Could you check a few things on this model? Use its own coordinates, in mm. Face numbers are marked on the shaded views. A direction names the side the tool comes from. Coordinates: 2 decimals unless noted, no trailing zeros. Loops run counter-clockwise (first coordinate to the right, second up) from the corner with the lowest first, then second, coordinate; pieces in that order, holes last.
1) Imagine slicing it at B-B on y = 5.5. Please give me the cut outline in (x, z), plus the area to 3 significant figures.
2) If I drill on line 1 along Z through (x, y) = (134.75, 45); line 2 along Z through (x, y) = (6.5, 2.5); line 3 along Y through (x, z) = (17, -90.7), over which ranges is the centre line in solid material (lowest first)?
3) Imagine slicing it at D-D on x = 123.5. Please give me the cut outline in (y, z).
4) Thinking about a two-plate mould opening in X: for the marked faces 6, 7 and 8, which applies, released by +X, released by -X, zero draft, split by the parting line, or undercut?
5) For the marked faces 1, 2, 3, 4 and 5, which set-ups out of +Z, -Z, +X, -X, +Y, -Y let a thin tool reach every point of the face, with its end or its side?
6) Will these pins go through, and if not, where does the flat tip stop? P1, Ø5, axis at y = 0.5, z = -75, coming from the -X side; P2, Ø4, axis at x = 12, y = 33.5, coming from the -Z side; P3, Ø13.5, axis at y = 16.5, z = -38.5, coming from the +X side; P4, Ø3, axis at x = -8.75, z = -96.14, coming from the +Y side.
7) Imagine slicing it at C-C on z = -84. Please give me the cut outline in (x, y).
8) Imagine slicing it at A-A on x = 17. Please give me the cut outline in (y, z), plus the area to 4 significant figures.
```python
from build123d import *

# Parameters (mm, degrees)
SKETCH1_W                = 136
SKETCH1_H                = 106
SKETCH1_W_2              = 126
SKETCH1_H_2              = 96
BOSS_EXTRUDE1_DEPTH      = 45
SKETCH2_W                = 136
SKETCH2_H                = 106
BOSS_EXTRUDE3_DEPTH      = 5
SKETCH3_R                = 10.5
CUT_EXTRUDE1_DEPTH       = 5
BOSS_EXTRUDE4_DEPTH      = 5
BOSS_EXTRUDE4_DEPTH_BACK = 5
SKETCH4_W                = 156
SKETCH4_H                = 126
SKETCH4_W_2              = 136
SKETCH4_H_2              = 106
SKETCH5_W                = 136
SKETCH5_H                = 106
SKETCH5_W_2              = 126
SKETCH5_H_2              = 96
BOSS_EXTRUDE6_DEPTH      = 5
CHAMFER1_SIZE            = 5
SKETCH6_R                = 1.75
CUT_EXTRUDE2_DEPTH       = 180.97284412


with BuildPart() as part:
    # Sketch1 → Boss-Extrude1 (new body)
    with BuildSketch(Plane(origin=(0, 0, 0), x_dir=(1, 0, 0), z_dir=(0, 1, 0))):
        with Locations((63, 39.392502756)):
            Rectangle(SKETCH1_W, SKETCH1_H)
        with Locations((63, 39.392502756)):
            Rectangle(SKETCH1_W_2, SKETCH1_H_2, mode=Mode.SUBTRACT)
    extrude(amount=BOSS_EXTRUDE1_DEPTH)

    # Sketch2 → Boss-Extrude3 (add)
    with BuildSketch(Plane.XZ):
        with Locations((63, -39.392502756)):
            Rectangle(SKETCH2_W, SKETCH2_H)
    extrude(amount=BOSS_EXTRUDE3_DEPTH)

    # Sketch3 → Cut-Extrude1 (cut)
    with BuildSketch(Plane.XY.offset(-87.392502756)):
        with Locations((17, 20)):
            Circle(SKETCH3_R)
    extrude(amount=-CUT_EXTRUDE1_DEPTH, mode=Mode.SUBTRACT)

    # Sketch4 → Boss-Extrude4 (add, two sides: drawn at the far end of the back side and taken through both)
    with BuildSketch(Plane(origin=(0, 45, 0), x_dir=(1, 0, 0), z_dir=(0, 1, 0)).offset(-BOSS_EXTRUDE4_DEPTH_BACK)):
        with Locations((63, 39.392502756)):
            Rectangle(SKETCH4_W, SKETCH4_H)
        with Locations((63, 39.392502756)):
            Rectangle(SKETCH4_W_2, SKETCH4_H_2, mode=Mode.SUBTRACT)
    extrude(amount=BOSS_EXTRUDE4_DEPTH + BOSS_EXTRUDE4_DEPTH_BACK)

    # Sketch5 → Boss-Extrude6 (add)
    with BuildSketch(Plane(origin=(0, 45, 0), x_dir=(1, 0, 0), z_dir=(0, 1, 0))):
        with Locations((63, 39.392502756)):
            Rectangle(SKETCH5_W, SKETCH5_H)
        with Locations((63, 39.392502756)):
            Rectangle(SKETCH5_W_2, SKETCH5_H_2, mode=Mode.SUBTRACT)
    extrude(amount=BOSS_EXTRUDE6_DEPTH)

    # Chamfer1
    chamfer1_edges = [part.edges().sort_by_distance(p)[0] for p in [
        (-15, 45, 23.607497244),
        (-15, 45, -102.392502756),
        (141, 45, -102.392502756),
        (141, 45, 23.607497244),
    ]]
    chamfer(chamfer1_edges, length=CHAMFER1_SIZE)

    # Sketch6 → Cut-Extrude2 (cut, through all)
    with BuildSketch(Plane.XZ.offset(-40)):
        with Locations(Location((-8.75, 17.357497244, 0), (0, 0, 270))):
            Circle(SKETCH6_R)
        with Locations(Location((-8.75, -96.142502756, 0), (0, 0, 90))):
            Circle(SKETCH6_R)
        with Locations(Location((134.75, -96.142502756, 0), (0, 0, 270))):
            Circle(SKETCH6_R)
        with Locations(Location((134.75, 17.357497244, 0), (0, 0, 90))):
            Circle(SKETCH6_R)
    extrude(amount=-CUT_EXTRUDE2_DEPTH, mode=Mode.SUBTRACT)


solid = part.part
```
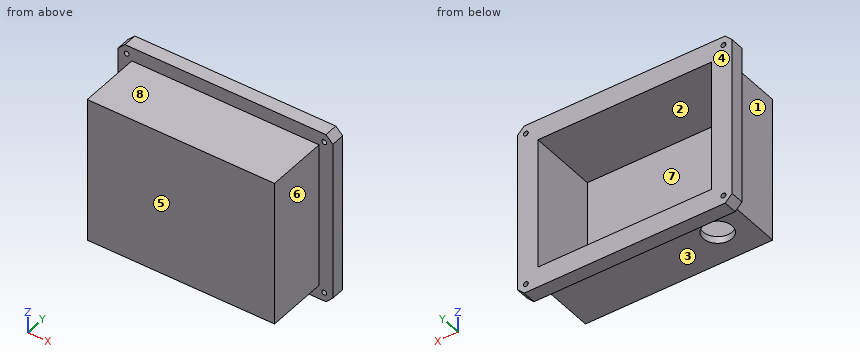
Filled in:
1. outline: (-5, -92.39) - (131, -92.39) - (131, 13.61) - (-5, 13.61) - close; hole (0, -87.39) - (126, -87.39) - (126, 8.61) - (0, 8.61) - close
1. area: 2,320 mm2
2. line 1: z = -102.39 to -97.89, -94.39 to 15.61, 19.11 to 23.61
2. line 2: z = -92.39 to -87.39, 8.61 to 13.61
2. line 3: y = -5 to 9.5, 30.5 to 50
3. outline: (-5, -92.39) - (40, -92.39) - (40, -102.39) - (50, -102.39) - (50, -87.39) - (0, -87.39) - (0, 8.61) - (50, 8.61) - (50, 23.61) - (40, 23.61) - (40, 13.61) - (-5, 13.61) - close
4. face 6: released by +X
4. face 7: undercut
4. face 8: zero draft
5. face 1: +Z, -Z, -X, -Y
5. face 2: +Y
5. face 3: -Z, +X, -X, -Y
5. face 4: +Z, -Z, +X, -X, +Y
5. face 5: +Z, -Z, +X, -X, -Y
6. P1: stops at x = -5
6. P2: stops at z = -92.39
6. P3: stops at x = 131
6. P4: passes through
7. outline: (-15, 40) - (-5, 40) - (-5, -5) - (131, -5) - (131, 40) - (141, 40) - (141, 50) - (126, 50) - (126, 0) - (0, 0) - (0, 50) - (-15, 50) - close
8. outline: (-5, -92.39) - (9.5, -92.39) - (9.5, -87.39) - (0, -87.39) - (0, 8.61) - (50, 8.61) - (50, 23.61) - (40, 23.61) - (40, 13.61) - (-5, 13.61) - close; (30.5, -92.39) - (40, -92.39) - (40, -102.39) - (50, -102.39) - (50, -87.39) - (30.5, -87.39) - close
8. area: 1,125 mm2
